from build123d import *

# Parameters (mm, degrees)
SKETCH_1_R          = 22.5
EXTRUDE_1_DEPTH     = 128
SKETCH_2_OUTSIDE_W  = 75.59
SKETCH_2_OUTSIDE_H  = 75.59
SKETCH_2_OUTSIDE_R  = 17.5
CUT_EXTRUDE_1_DEPTH = 23
SKETCH_3_OUTSIDE_W  = 75.59
SKETCH_3_OUTSIDE_H  = 75.59
SKETCH_3_OUTSIDE_R  = 20
CUT_EXTRUDE_2_DEPTH = 74
SKETCH_4_OUTSIDE_W  = 75.59
SKETCH_4_OUTSIDE_H  = 75.59
SKETCH_4_OUTSIDE_R  = 17.5
CUT_EXTRUDE_3_DEPTH = 23
CUT_EXTRUDE_START   = 15.5
CUT_EXTRUDE_4_DEPTH = 117.3957922
CHAMFER_1_SIZE      = 2


with BuildPart() as part:
    # 草图1 → 凸台-拉伸1 (new body)
    with BuildSketch(Plane(origin=(0, 0, 0), x_dir=(0, 0, -1), z_dir=(1, 0, 0))):
        Circle(SKETCH_1_R)
    extrude(amount=EXTRUDE_1_DEPTH)

    # 草图2 outside → 切除-拉伸1 (cut)
    with BuildSketch(Plane(origin=(128, 0, 0), x_dir=(0, 0, -1), z_dir=(1, 0, 0))):
        Rectangle(SKETCH_2_OUTSIDE_W, SKETCH_2_OUTSIDE_H)
        Circle(SKETCH_2_OUTSIDE_R, mode=Mode.SUBTRACT)
    extrude(amount=-CUT_EXTRUDE_1_DEPTH, mode=Mode.SUBTRACT)

    # 草图3 outside → 切除-拉伸2 (cut)
    with BuildSketch(Plane.ZY):
        Rectangle(SKETCH_3_OUTSIDE_W, SKETCH_3_OUTSIDE_H)
        Circle(SKETCH_3_OUTSIDE_R, mode=Mode.SUBTRACT)
    extrude(amount=-CUT_EXTRUDE_2_DEPTH, mode=Mode.SUBTRACT)

    # 草图4 outside → 切除-拉伸3 (cut)
    with BuildSketch(Plane.ZY):
        Rectangle(SKETCH_4_OUTSIDE_W, SKETCH_4_OUTSIDE_H)
        with Locations(Location((0, 0, 0), (0, 0, 180))):
            Circle(SKETCH_4_OUTSIDE_R, mode=Mode.SUBTRACT)
    extrude(amount=-CUT_EXTRUDE_3_DEPTH, mode=Mode.SUBTRACT)

    # 草图5 → 切除-拉伸4 (cut, through all)
    with BuildSketch(Plane.XY.offset(CUT_EXTRUDE_START)):
        with BuildLine():
            Line((30.362609491, 4.362609491), (66.637390509, 4.362609491))
            ThreePointArc((66.637390509, 4.362609491), (71, 0), (66.637390509, -4.362609491))
            Line((66.637390509, -4.362609491), (30.362609491, -4.362609491))
            ThreePointArc((30.362609491, -4.362609491), (26, 0), (30.362609491, 4.362609491))
        make_face()
    extrude(amount=CUT_EXTRUDE_4_DEPTH, mode=Mode.SUBTRACT)

    # 倒角1
    chamfer_1_edges = [part.edges().sort_by_distance(p)[0] for p in [
        (128, 0, 17.5),
        (0, 0, 17.5),
    ]]
    chamfer(chamfer_1_edges, length=CHAMFER_1_SIZE)


solid = part.part
Part model, mm, in its own coordinate system. A direction names the side the tool comes from. Coordinates: 2 decimals unless noted, no trailing zeros. Loops run counter-clockwise (first coordinate to the right, second up) from the corner with the lowest first, then second, coordinate; pieces in that order, holes last. Notation, with made-up numbers: M 38.25,43.5 L 61.25,43.5 A14 cw 61.25,64.5 Z; hole C 25.25,-37.75 d8. An arc over 180 degrees is marked long. Use a Markdown table: item, result. Add a question column.
Q1. Which spindle directions (+Z, -Z, +X, -X, +Y, -Y) get a long thin tool onto all of the face, cutting with end or side? Do faces 4 (the cylindrical face through (26, 0, 18)), 5 (the cylindrical face through (89.283, -19.961, -10.382)), 6 (the flat face through (128, 0, 0)), 7 (the cylindrical face through (115.647, -10.648, 13.887)), 8 (the cylindrical face through (48.143, -19.524, -4.336)). Say none if no direction does.
Q2. Cut at D-D (x = 95.5). Write the cut outline in (y, z).
Q3. Probe L1, parallel to X at y = 13, z = -14.5; L2, parallel to Y at x = 28, z = -1; L3, parallel to Y at x = 30, z = -3.5. List the from-to ranges inside material, lowest first.
Q4. Cut at B-B (z = 0). Write the cut outline in (x, y), and give its area (3 significant figures).
Q5. Cut at A-A (y = 0). Write the cut outline in (x, z).
Q6. Cut at C-C (x = 120). Write the cut outline in (y, z).
Q7. Mould opens along Y. For faces 1 (the flat face through (0, 0, 0)), 2 (the flat face through (49, 0, 15.5)), 3 (the cylindrical face through (12.353, 17.084, 3.794)) say: +Y half, -Y half, draft (parallel to the pull), parting line (faces both ways), or undercut.
Q8. Pin check, flat tips, straight feed: P1, Ø2, axis at x = 48.5, z = 17, coming from the +Y side; P2, Ø3, axis at y = -8.5, z = 17.5, coming from the -X side; P3, Ø5, axis at x = 84.5, z = 4.5, coming from the -Y side. Stop position of each tip, or through.
Worked out:
| question | item | result |
|---|---|---|
| 1 | face 4 | +Z |
| 1 | face 5 | +X, -X |
| 1 | face 6 | +Z, -Z, +X, +Y, -Y |
| 1 | face 7 | +X |
| 1 | face 8 | -X |
| 2 | outline | C 0,0 d45 |
| 3 | L1 | x = 23 to 105 |
| 3 | L2 | y = -19.97 to 19.97 |
| 3 | L3 | y = -19.69 to 19.69 |
| 4 | outline | M 0,-15.5 L 2,-17.5 L 23,-17.5 L 23,-20 L 74,-20 L 74,-22.5 L 105,-22.5 L 105,-17.5 L 126,-17.5 L 128,-15.5 L 128,15.5 L 126,17.5 L 105,17.5 L 105,22.5 L 74,22.5 L 74,20 L 23,20 L 23,17.5 L 2,17.5 L 0,15.5 Z |
| 4 | area | 5,040 mm2 |
| 5 | outline | M 0,-15.5 L 2,-17.5 L 23,-17.5 L 23,-20 L 74,-20 L 74,-22.5 L 105,-22.5 L 105,-17.5 L 126,-17.5 L 128,-15.5 L 128,15.5 L 126,17.5 L 105,17.5 L 105,22.5 L 74,22.5 L 74,20 L 71,20 L 71,15.5 L 26,15.5 L 26,20 L 23,20 L 23,17.5 L 2,17.5 L 0,15.5 Z |
| 6 | outline | C 0,0 d35 |
| 7 | face 1 | draft |
| 7 | face 2 | undercut |
| 7 | face 3 | parting line |
| 8 | P1 | stops at y = 12 |
| 8 | P2 | stops at x = 23 |
| 8 | P3 | stops at y = -22.41 |
